```python
from build123d import *

# Parameters (mm, degrees)
F0_R     = 1.5875
F1_DEPTH = 3.175
F2_DEPTH = 1.524
F4_DEPTH = 3.175
F5_R     = 2.032
F6_SIZE2 = 1.27
F6_SIZE  = 2.286


with BuildPart() as f1:
    # F0 (on Top) → F1 (new body)
    with BuildSketch(Plane.XY):
        with BuildLine():
            Line((-9.6292242988, 40.124001728), (0.2798453521, 40.124001728))
            Line((0.2798453521, 40.124001728), (10.1889150029, 40.124001728))
            Line((10.1889150029, 40.124001728), (12.9798453521, 40.124001728))
            Line((12.9798453521, 40.124001728), (12.9798453521, 36.9588285685))
            Line((12.9798453521, 36.9588285685), (12.9798453521, 14.724001728))
            Line((12.9798453521, 14.724001728), (25.6798453521, 14.724001728))
            Line((25.6798453521, 14.724001728), (25.6798453521, 52.824001728))
            Line((25.6798453521, 52.824001728), (9.8048453521, 52.824001728))
            ThreePointArc((9.8048453521, 52.824001728), (0.2798453521, 43.299001728), (-9.2451546479, 52.824001728))
            Line((-9.2451546479, 52.824001728), (-25.1201546479, 52.824001728))
            Line((-25.1201546479, 52.824001728), (-25.1201546479, 14.724001728))
            Line((-25.1201546479, 14.724001728), (-12.4201546479, 14.724001728))
            Line((-12.4201546479, 14.724001728), (-12.4201546479, 36.9588285685))
            Line((-12.4201546479, 36.9588285685), (-12.4201546479, 40.124001728))
            Line((-12.4201546479, 40.124001728), (-9.6292242988, 40.124001728))
        make_face()
        Polygon((10.1889150029, 40.124001728), (0.2798453521, 40.124001728), (-9.6292242988, 40.124001728), (-12.4201546479, 40.124001728), (-12.4201546479, 36.9588285685), (-9.5826818713, 36.9588285685), (0.2798453521, 36.9588285685), (12.9798453521, 36.9588285685), (12.9798453521, 40.124001728), align=None)
        Polygon((12.9798453521, 14.724001728), (12.9798453521, 36.9588285685), (0.2798453521, 36.9588285685), (-9.5826818713, 36.9588285685), (-12.4201546479, 36.9588285685), (-12.4201546479, 14.724001728), align=None)
        with Locations((0.2798453521, 33.3929099143)):
            Circle(F0_R, mode=Mode.SUBTRACT)
        with Locations((0.2798453521, 33.3929099143)):
            Circle(F0_R)
    extrude(amount=-F1_DEPTH)

    # F0 (on Top) → F2 (join)
    with BuildSketch(Plane.XY):
        with BuildLine():
            Line((-9.6292242988, 40.124001728), (0.2798453521, 40.124001728))
            Line((0.2798453521, 40.124001728), (10.1889150029, 40.124001728))
            Line((10.1889150029, 40.124001728), (12.9798453521, 40.124001728))
            Line((12.9798453521, 40.124001728), (12.9798453521, 36.9588285685))
            Line((12.9798453521, 36.9588285685), (12.9798453521, 14.724001728))
            Line((12.9798453521, 14.724001728), (25.6798453521, 14.724001728))
            Line((25.6798453521, 14.724001728), (25.6798453521, 52.824001728))
            Line((25.6798453521, 52.824001728), (9.8048453521, 52.824001728))
            ThreePointArc((9.8048453521, 52.824001728), (0.2798453521, 43.299001728), (-9.2451546479, 52.824001728))
            Line((-9.2451546479, 52.824001728), (-25.1201546479, 52.824001728))
            Line((-25.1201546479, 52.824001728), (-25.1201546479, 14.724001728))
            Line((-25.1201546479, 14.724001728), (-12.4201546479, 14.724001728))
            Line((-12.4201546479, 14.724001728), (-12.4201546479, 36.9588285685))
            Line((-12.4201546479, 36.9588285685), (-12.4201546479, 40.124001728))
            Line((-12.4201546479, 40.124001728), (-9.6292242988, 40.124001728))
        make_face()
    extrude(amount=F2_DEPTH)

    # F3 (on face) → F4 (join)
    with BuildSketch(Plane.XY.offset(1.524)):
        with BuildLine():
            Line((-25.1201546479, 14.724001728), (-12.4201546479, 14.724001728))
            Line((-12.4201546479, 14.724001728), (-12.4201546479, 36.9455851614))
            Line((-12.4201546479, 36.9455851614), (-12.4201546479, 40.124001728))
            Line((-12.4201546479, 40.124001728), (0.2798453521, 40.124001728))
            Line((0.2798453521, 40.124001728), (12.9798453521, 40.124001728))
            Line((12.9798453521, 40.124001728), (12.9798453521, 36.9455851614))
            Line((12.9798453521, 36.9455851614), (12.9798453521, 14.724001728))
            Line((12.9798453521, 14.724001728), (25.6798453521, 14.724001728))
            Line((25.6798453521, 14.724001728), (25.6798453521, 52.824001728))
            Line((25.6798453521, 52.824001728), (9.8048453521, 52.824001728))
            ThreePointArc((9.8048453521, 52.824001728), (0.2798453521, 43.299001728), (-9.2451546479, 52.824001728))
            Line((-9.2451546479, 52.824001728), (-25.1201546479, 52.824001728))
            Line((-25.1201546479, 52.824001728), (-25.1201546479, 14.724001728))
        make_face()
        Polygon((-12.4201546479, 36.9455851614), (-12.4201546479, 14.724001728), (12.9798453521, 14.724001728), (12.9798453521, 36.9455851614), (0.2798453521, 36.9455851614), align=None)
        with BuildLine():
            ThreePointArc((1.8673453521, 33.7810702622), (-0.8426866631, 32.6585382471), (0.2798453521, 35.3685702622))
            ThreePointArc((0.2798453521, 35.3685702622), (1.4023773672, 34.9036022773), (1.8673453521, 33.7810702622))
        make_face(mode=Mode.SUBTRACT)
    extrude(amount=F4_DEPTH)

    # F5
    f5_edges = [f1.edges().sort_by_distance(p)[0] for p in [
        (0.279845, 14.724002, 1.524),
        (0.279845, 14.724002, 0),
        (-12.420155, 14.724002, 0.762),
        (12.979845, 14.724002, 0.762),
    ]]
    fillet(f5_edges, radius=F5_R)

    # F6
    f6_edges = [f1.edges().sort_by_distance(p)[0] for p in [
        (0.279845, 32.19357, 4.699),
    ]]
    f6_side = f1.faces().sort_by_distance((0.279845, 32.19357, 3.1115))[0]
    chamfer(f6_edges, length=F6_SIZE, length2=F6_SIZE2, reference=f6_side)


solid = f1.part
```
Design review of the part built by this model. Coordinates are the model's own, in mm. A direction names the side the tool comes from. Give positions to 0.01 mm unless a question says otherwise; leave off trailing zeros. Write each loop counter-clockwise with the first axis right and the second up, starting at its lowest first coordinate (ties: lowest second). Pieces come first, ordered by that corner, then holes.
(1) Wall thickness on line 1 along Z through (x, y) = (-4, 18) (3 decimals); line 2 along Y through (x, z) = (-11, 1.75); line 3 along Y through (x, z) = (0, 1.25): over which ranges is each line inside the solid? List them lowest first.
Checked values:
line 1: z = -3.175 to 0, 1.524 to 4.699
line 2: y = 15.82 to 36.95, 40.12 to 52.82
line 3: y = 40.12 to 43.3
(2) Clearance check with flat-ended pins moving along their axes: pin 1 Ø2.5 at (x, z) = (0, 3) entering from -Y; pin 2 Ø3 at (x, z) = (7.5, 1.5) entering from -Y; pin 3 Ø1.6 at (x, z) = (5.5, 3) entering from +Y. State where each tip first meets the part, or that it passes through.
Checked values:
pin 1: stops at y = 14.72
pin 2: stops at y = 14.8
pin 3: stops at y = 45.44
(3) Add section C-C (z = 3). Give the boundary of the cut face in (x, y) (3 decimals).
Checked values:
outline: (-25.12, 14.724) - (-14.452, 14.724) arc R2.032 ccw to (-13.896, 14.802) - (14.456, 14.802) arc R2.032 ccw to (15.012, 14.724) - (25.68, 14.724) - (25.68, 52.824) - (9.805, 52.824) arc R9.525 cw to (-9.245, 52.824) - (-25.12, 52.824) - close; hole (-12.42, 36.946) - (12.98, 36.946) - (12.98, 40.124) - (-12.42, 40.124) - close; hole circle Ø3.827 at (0.28, 33.781)
(4) Tool access review of faces 1 (the face through (12.98, 31, 1)), 2 (the face through (0, 29, 0)), 3 (the face through (0, 40.124, 2)): name each direction out of +Z, -Z, +X, -X, +Y, -Y from which nothing blocks a thin tool from reaching the whole face with its end or side.
Checked values:
face 1: none
face 2: -Y
face 3: +Z
(5) Add section D-D (z = -1.5). Give the boundary of the cut face in (x, y) (3 decimals), and give its area (3 significant figures).
Checked values:
outline: (-25.12, 14.724) - (-14.452, 14.724) arc R2.032 ccw to (-13.92, 14.795) - (14.48, 14.795) arc R2.032 ccw to (15.012, 14.724) - (25.68, 14.724) - (25.68, 52.824) - (9.805, 52.824) arc R9.525 cw to (-9.245, 52.824) - (-25.12, 52.824) - close
area: 1,790 mm2
(6) Mouldability with a two-part tool opening along X and no side actions: class faces 4 (the face through (0, 34, -3.175)), 5 (the face through (-13.305, 15.079, 0.801)), 6 (the face through (25.68, 34, 1)) as +X half, -X half, draft (parallel to the pull), parting line (faces both ways), or undercut.
Checked values:
face 4: draft
face 5: undercut
face 6: +X half
(7) Add section A-A (y = 27). Give the boundary of the cut face in (x, z) (3 decimals).
Checked values:
outline: (-25.12, -3.175) - (25.68, -3.175) - (25.68, 4.699) - (-25.12, 4.699) - close; hole (-12.42, 0) - (12.98, 0) - (12.98, 1.524) - (-12.42, 1.524) - close
(8) Add section B-B (y = 45). Give the boundary of the cut face in (x, z) (3 decimals), and give its area (3 significant figures).
Checked values:
outline: (-25.12, -3.175) - (-5.153, -3.175) - (-5.153, 4.699) - (-25.12, 4.699) - close; (5.712, -3.175) - (25.68, -3.175) - (25.68, 4.699) - (5.712, 4.699) - close
area: 314 mm2
